```python
from build123d import *

# Parameters (mm, degrees)
F0_R     = 27
F1_DEPTH = 10
F2_R     = 14.65
F3_DEPTH = 25
F4_R     = 12.2
F5_DEPTH = 25
F6_R     = 3
F7_DEPTH = 5


with BuildPart() as f1:
    # F0 (on Top) → F1 (new body)
    with BuildSketch(Plane.XY):
        Circle(F0_R)
    extrude(amount=F1_DEPTH)

    # F2 (on face) → F3 (join)
    with BuildSketch(Plane.XY.offset(10)):
        Circle(F2_R)
    extrude(amount=F3_DEPTH)

    # F4 (on face) → F5 (cut)
    with BuildSketch(Plane.XY.offset(35)):
        Circle(F4_R)
    extrude(amount=-F5_DEPTH, mode=Mode.SUBTRACT)

    # F6 (on face) → F7 (cut)
    with BuildSketch(Plane.XY.offset(10)):
        Circle(F6_R)
    extrude(amount=-F7_DEPTH, mode=Mode.SUBTRACT)


solid = f1.part
```
Geometry check sheet. Reference: the model listing, model coordinates, mm. A direction names the side the tool comes from. Coordinates: 2 decimals unless noted, no trailing zeros. Order: outer loops, then holes, each group sorted by start corner. A loop starts at its lowest first (then second) coordinate and runs counter-clockwise, first axis right, second up. Notation, with made-up numbers: (12, 63) - (56, 63) arc R28 ccw to (56, 101) - close; hole circle Ø1 at (34.5, 53). An arc over 180 degrees is marked (long way). Use one line per item in the form item = value.
1. Section check C-C (z = 13.5). Record the boundary of the cut face in (x, y), then the cut area to 3 significant figures.
Here are the results:
outline = circle Ø29.3 at (0, 0); hole circle Ø24.4 at (0, 0)
area = 207 mm²
2. Gauge pin test, flat ends, axial feed: pin 1 (1.8 mm diameter, centred on x = 1, y = 1.5, fed in from +Z); pin 2 (9.5 mm diameter, centred on x = 0, y = 0, fed in from +Z); pin 3 (4 mm diameter, centred on x = 12, z = 16, fed in from -Y). Record the tip position at first contact, or that the pin passes through.
Here are the results:
pin_1 = 5
pin_2 = 10
pin_3 = -10.71
3. Draft check along Y on faces 3 (the face through (-12.19, 0.54, 22.68)), 4 (the face through (13.973, 4.4, 22.325)), 5 (the face through (12, -12, 10)). Enter one of: pulls with the +Y half, pulls with the -Y half, needs draft (parallel to the pull), parting line crosses it, or undercut.
Here are the results:
face_3 = undercut
face_4 = parting line crosses it
face_5 = needs draft
4. Access from +Z, -Z, +X, -X, +Y, -Y to the whole of each face (thin tool, end or side, straight path). Record for faces 1 (the face through (-3, 12, 35)), 2 (the face through (0, 0, 5)).
Here are the results:
face_1 = +Z, +X, -X, +Y, -Y
face_2 = +Z
5. Scan lines: line 1 (Y direction, x = 0, z = 22); line 2 (Z direction, x = 5.5, y = 6); line 3 (X direction, y = 1, z = 6). Record each from-to range of solid material in increasing order.
Here are the results:
line_1 = -14.65 to -12.2, 12.2 to 14.65
line_2 = 0 to 10
line_3 = -26.98 to -2.83, 2.83 to 26.98
6. Section check D-D (z = 3.5). Record the boundary of the cut face in (x, y), then the cut area to 3 significant figures.
Here are the results:
outline = circle Ø54 at (0, 0)
area = 2,290 mm²
7. Section check A-A (x = 0). Record the boundary of the cut face in (y, z), then the cut area to 4 significant figures.
Here are the results:
outline = (-27, 0) - (27, 0) - (27, 10) - (14.65, 10) - (14.65, 35) - (12.2, 35) - (12.2, 10) - (3, 10) - (3, 5) - (-3, 5) - (-3, 10) - (-12.2, 10) - (-12.2, 35) - (-14.65, 35) - (-14.65, 10) - (-27, 10) - close
area = 632.5 mm²
